Geometry: final body of the model. Coordinates: model frame, mm. Coordinates: 2 decimals unless noted, no trailing zeros. Order: outer loops, then holes, each group sorted by start corner. A loop starts at its lowest first (then second) coordinate and runs counter-clockwise, first axis right, second up. Notation, with made-up numbers: (86, 6.5) - (105, 6.5) arc R30 cw to (105, 44.5) - close; hole circle Ø11 at (-31, 36.25). An arc over 180 degrees is marked (long way). Use one line per item in the form item = value. Start each with the question number.
```python
from build123d import *

# Parameters (mm, degrees)
SKETCH1_R               = 30
SKETCH1_R_2             = 28
BOSS_EXTRUDE1_DEPTH     = 708
SKETCH2_R               = 5
CUT_EXTRUDE1_DEPTH      = 31
CUT_EXTRUDE1_DEPTH_BACK = 31


with BuildPart() as part:
    # Sketch1 → Boss-Extrude1 (new body)
    with BuildSketch(Plane.XY):
        Circle(SKETCH1_R)
        Circle(SKETCH1_R_2, mode=Mode.SUBTRACT)
    extrude(amount=BOSS_EXTRUDE1_DEPTH)

    # Sketch2 → Cut-Extrude1 (cut, two sides)
    with BuildSketch(Plane(origin=(0, 0, 0), x_dir=(1, 0, 0), z_dir=(0, 1, 0))) as cut_extrude1_sk:
        with Locations((0, -683)):
            Circle(SKETCH2_R)
        with Locations((0, -25)):
            Circle(SKETCH2_R)
    extrude(amount=CUT_EXTRUDE1_DEPTH, mode=Mode.SUBTRACT)
    extrude(cut_extrude1_sk.sketch, amount=-CUT_EXTRUDE1_DEPTH_BACK, mode=Mode.SUBTRACT)


solid = part.part
```
(1) Cut plane B-B on x = -16. Return the cut outline in (y, z).
(2) Contact query for flat-ended pins moving along their axis: pin 1 Ø4 at (y, z) = (13, 355.5) entering from -X; pin 2 Ø10 at (y, z) = (11.5, 85.5) entering from +X; pin 3 Ø2 at (y, z) = (-12.5, 94) entering from -X. Output: stop coordinate, or through.
(3) Cut plane A-A on y = 0. Return the cut outline in (x, z).
(4) Draft query along Y for faces 1 (the cylindrical face through (25.865, -10.724, 349.044)), 2 (the flat face through (-25, 13, 708)), 3 (the cylindrical face through (-29.97, 1.32, 349.04)). Return one class per face: released by +Y, released by -Y, zero draft, split by the parting line, or undercut.
(5) Material intervals for L1, parallel to Z at x = 0, y = 29.05; L2, parallel to X at y = 1.5, z = 170.5; L3, parallel to Y at x = -0.5, z = 199.5, sorted ascending. Write a range as from..to.
(6) Cut plane C-C on z = 586.5. Return the cut outline in (x, y).
Check sheet entries:
q1.outline = (-25.38, 0) - (-22.98, 0) - (-22.98, 708) - (-25.38, 708) - close; (22.98, 0) - (25.38, 0) - (25.38, 708) - (22.98, 708) - close
q2.pin_1 = -27.91
q2.pin_2 = 29.29
q2.pin_3 = -27.71
q3.outline = (-30, 0) - (-28, 0) - (-28, 708) - (-30, 708) - close; (28, 0) - (30, 0) - (30, 708) - (28, 708) - close
q4.face_1 = undercut
q4.face_2 = zero draft
q4.face_3 = split by the parting line
q5.L1 = 0..20, 30..678, 688..708
q5.L2 = -29.96..-27.96, 27.96..29.96
q5.L3 = -30..-28, 28..30
q6.outline = circle Ø60 at (0, 0); hole circle Ø56 at (0, 0)
